For this review, take the finished solid that the model builds, in its own axes (mm). Give positions to 0.01 mm unless a question says otherwise; leave off trailing zeros. Loops run counter-clockwise (first coordinate to the right, second up) from the corner with the lowest first, then second, coordinate; pieces in that order, holes last. Notation, with made-up numbers: (-28, -17) - (-1, -17) arc R34 ccw to (-1, 17) - close; hole circle Ø6 at (69.5, 33). An arc over 180 degrees is marked (long way). Answer in a Markdown table with one row per item.
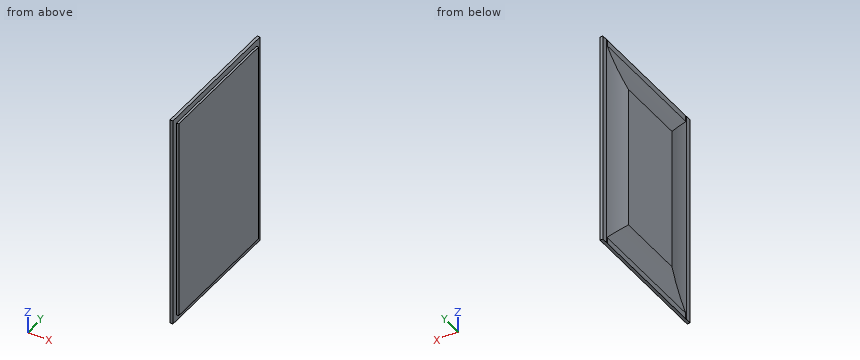
```python
from build123d import *

# Parameters (mm, degrees)
F0_W     = 304.8
F0_H     = 457.2
F1_DEPTH = 19.05
F2_W     = 4.7625
F2_H     = 12.7
F3_DEPTH = 457.201
F4_W     = 4.7625
F4_H     = 12.7
F5_DEPTH = 304.801


with BuildPart() as f1:
    # F0 (on Right) → F1 (new body)
    with BuildSketch(Plane.YZ):
        with Locations((-152.4, 228.6)):
            Rectangle(F0_W, F0_H)
    extrude(amount=F1_DEPTH)

    # F2 (on face) → F3 (cut, through all)
    with BuildSketch(Plane(origin=(0, 0, 0), x_dir=(1, 0, 0), z_dir=(0, 0, -1))):
        with Locations((16.66875, 6.35)):
            Rectangle(F2_W, F2_H)
        with Locations((16.66875, 298.45)):
            Rectangle(F2_W, F2_H)
        with BuildLine():
            Line((0, 0), (7.9375, 0))
            Line((7.9375, 0), (7.9375, 12.7))
            ThreePointArc((7.9375, 12.7), (6.046964, 44.709777), (0, 76.2))
            Line((0, 76.2), (0, 0))
        make_face()
        with BuildLine():
            Line((0, 304.8), (0, 228.6))
            ThreePointArc((0, 228.6), (6.046964, 260.090223), (7.9375, 292.1))
            Line((7.9375, 292.1), (7.9375, 304.8))
            Line((7.9375, 304.8), (0, 304.8))
        make_face()
    extrude(amount=-F3_DEPTH, mode=Mode.SUBTRACT)

    # F4 (on face) → F5 (cut, through all)
    with BuildSketch(Plane(origin=(0, 0, 0), x_dir=(-1, 0, 0), z_dir=(0, 1, 0))):
        with BuildLine():
            Line((0, 457.2), (-7.9375, 457.2))
            Line((-7.9375, 457.2), (-7.9375, 444.5))
            ThreePointArc((-7.9375, 444.5), (-5.945434, 412.502915), (0, 381))
            Line((0, 381), (0, 457.2))
        make_face()
        with BuildLine():
            Line((-7.9375, 12.7), (-7.9375, 0))
            Line((-7.9375, 0), (0, 0))
            Line((0, 0), (0, 76.2))
            ThreePointArc((0, 76.2), (-5.945434, 44.697085), (-7.9375, 12.7))
        make_face()
        with Locations((-16.66875, 450.85)):
            Rectangle(F4_W, F4_H)
        with Locations((-16.66875, 6.35)):
            Rectangle(F4_W, F4_H)
    extrude(amount=-F5_DEPTH, mode=Mode.SUBTRACT)


solid = f1.part
```
1. We need section A-A, the plane y = -203. Give the boundary of the cut face in (x, z), and give its area (3 significant figures).
Values:
| item | result |
|---|---|
| outline | (0, 76.2) arc R257.97 cw to (7.94, 12.7) - (7.94, 0) - (14.29, 0) - (14.29, 12.7) - (19.05, 12.7) - (19.05, 444.5) - (14.29, 444.5) - (14.29, 457.2) - (7.94, 457.2) - (7.94, 444.5) arc R257.97 cw to (0, 381) - close |
| area | 7,710 mm^2 |
2. We need section C-C, the plane x = 5. Give the boundary of the cut face in (y, z), and give its area (3 significant figures).
Values:
| item | result |
|---|---|
| outline | (-252.64, 51.52) - (-52.16, 51.52) - (-52.16, 405.68) - (-252.64, 405.68) - close |
| area | 71,000 mm^2 |
3. Wall thickness on line 1 (Z direction, x = 14.5, y = -167.5); line 2 (Y direction, x = 17, z = 137.5); line 3 (X direction, y = -239, z = 142.5): over which ranges is each line inside the solid? List them lowest first. Write a range as [from, to].
Values:
| item | result |
|---|---|
| line 1 | z = [12.7, 444.5] |
| line 2 | y = [-292.1, -12.7] |
| line 3 | x = [2.47, 19.05] |
4. Clearance check with flat-ended pins moving along their axes: pin 1 (6 mm diameter, centred on x = 10.5, y = -87, fed in from -Z); pin 2 (14 mm diameter, centred on y = -5, z = 303, fed in from -X); pin 3 (1 mm diameter, centred on x = 16.5, z = 209.5, fed in from +Y); pin 4 (1.4 mm diameter, centred on x = 17.5, z = 122.5, fed in from -Y). State where each tip first meets the part, or that it passes through.
Values:
| item | result |
|---|---|
| pin 1 | stops at z = 0 |
| pin 2 | stops at x = 7.94 |
| pin 3 | stops at y = -12.7 |
| pin 4 | stops at y = -292.1 |
5. We need section B-B, the plane z = 118.5. Give the boundary of the cut face in (x, y), and give its area (3 significant figures).
Values:
| item | result |
|---|---|
| outline | (0, -228.6) arc R245.47 cw to (7.94, -292.1) - (7.94, -304.8) - (14.29, -304.8) - (14.29, -292.1) - (19.05, -292.1) - (19.05, -12.7) - (14.29, -12.7) - (14.29, 0) - (7.94, 0) - (7.94, -12.7) arc R245.47 cw to (0, -76.2) - close |
| area | 4,800 mm^2 |
